Source: CAD feature listing. Evaluate the final solid. Frame: model axes, mm. Face numbers are marked on the shaded views. A direction names the side the tool comes from. Round coordinates to 2 decimals unless told otherwise and drop trailing zeros. Loops run counter-clockwise (first coordinate to the right, second up) from the corner with the lowest first, then second, coordinate; pieces in that order, holes last.
(1) Set-up query: the marked faces 4, 5, 6, 7 and 8. Return all of +Z, -Z, +X, -X, +Y, -Y with unobstructed straight access to the full face (end or side cutting, diameter ignored); none if empty.
(2) First-contact query: pin 1 Ø2.5 at (x, z) = (-24.9, 3.5) entering from +Y; pin 2 Ø3.5 at (x, z) = (-25.5, 3) entering from +Y. Flat tips, straight axial feed; report the tip coordinate or a pass-through.
(3) Section B-B, the plane y = 19.5. Return the cut outline in (x, z), plus the area to 3 significant figures.
(4) Mould query, pull axis X, two halves, no side actions, for the marked faces 1, 2 and 3. Classes: pulls with the +X half, pulls with the -X half, needs draft (parallel to the pull), parting line crosses it, or undercut.
(5) Section C-C, the plane x = 13.5. Return the cut outline in (y, z), plus the area to 3 significant figures.
(6) Material intervals for probe 1 along Y at (x, z) = (22.5, 4.75); probe 2 along Z at (x, y) = (-24.9, -3.75); probe 3 along X at (y, z) = (-12.5, 4.25), sorted ascending.
(7) Section A-A, the plane z = 4.25. Return the cut outline in (x, y).
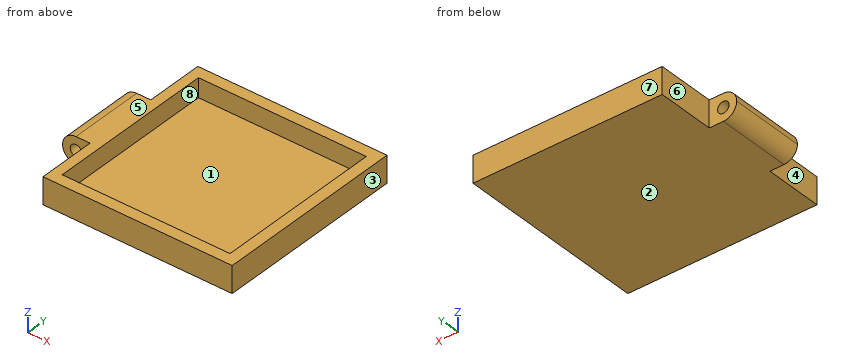
```python
from build123d import *

# Parameters (mm, degrees)
F1_DEPTH = 7
F2_R     = 3.49999
F4_D     = 3
F5_W     = 44
F5_H     = 44
F6_DEPTH = 5


# Not quite as in the source:
# - a fillet or chamfer is up to 0.001 mm smaller than in the source, because OpenCascade refuses the exact size


with BuildPart() as f1:
    # F0 (on Top) → F1 (new body)
    with BuildSketch(Plane.XY):
        Polygon((28.4, 25), (-21.2, 25), (-21.2, 9.8), (-28.4, 9.8), (-28.4, -9.8), (-21.2, -9.8), (-21.2, -25), (28.4, -25), align=None)
    extrude(amount=F1_DEPTH)

    # F2 (radius 3.5 in the source; OpenCascade refuses exactly that, so slightly less here)
    f2_edges = [f1.edges().sort_by_distance(p)[0] for p in [
        (-28.4, 0, 7),
        (-28.4, 0, 0),
    ]]
    fillet(f2_edges, radius=F2_R)

    # F4 (through all)
    with Locations(Plane(origin=(0, 9.8, 0), x_dir=(-1, 0, 0), z_dir=(0, 1, 0))):
        with Locations((24.9, 3.5)):
            Hole(F4_D / 2)

    # F5 (on face) → F6 (cut)
    with BuildSketch(Plane.XY.offset(7)):
        with Locations((3.4, 0)):
            Rectangle(F5_W, F5_H)
    extrude(amount=-F6_DEPTH, mode=Mode.SUBTRACT)


solid = f1.part
```
Output values:
1. face 4: +Z, -Z, -X, -Y
1. face 5: +Z, +X, -X, +Y, -Y
1. face 6: +Z, -Z, -X, +Y
1. face 7: +Z, -Z, +X, -X, +Y
1. face 8: +Z
2. pin 1: passes through
2. pin 2: stops at y = 9.8
3. outline: (-21.2, 0) - (28.4, 0) - (28.4, 7) - (25.4, 7) - (25.4, 2) - (-18.6, 2) - (-18.6, 7) - (-21.2, 7) - close
3. area: 127 mm2
4. face 1: undercut
4. face 2: needs draft
4. face 3: pulls with the +X half
5. outline: (-25, 0) - (25, 0) - (25, 7) - (22, 7) - (22, 2) - (-22, 2) - (-22, 7) - (-25, 7) - close
5. area: 130 mm2
6. probe 1: y = -25 to -22, 22 to 25
6. probe 2: z = 0 to 2, 5 to 7
6. probe 3: x = -21.2 to -18.6, 25.4 to 28.4
7. outline: (-28.32, -9.8) - (-26.2, -9.8) - (-26.2, 9.8) - (-28.32, 9.8) - close; (-23.6, -9.8) - (-21.2, -9.8) - (-21.2, -25) - (28.4, -25) - (28.4, 25) - (-21.2, 25) - (-21.2, 9.8) - (-23.6, 9.8) - close; hole (-18.6, -22) - (25.4, -22) - (25.4, 22) - (-18.6, 22) - close
